Can you work these out from the model? Positions are in its coordinate system, mm. A direction names the side the tool comes from. Coordinates: 2 decimals unless noted, no trailing zeros. Loops run counter-clockwise (first coordinate to the right, second up) from the corner with the lowest first, then second, coordinate; pieces in that order, holes last. Notation, with made-up numbers: (83, -22.5) -> (92, -22.5) arc R9 cw to (92, -14.5) -> close; hole circle Ø4 at (70.5, 47.25). An arc over 180 degrees is marked (long way). Use one line per item in the form item = value. Start each with the question number.
(1) I need wall thicknesses on line 1 (X direction, y = -1.65, z = 0); line 2 (Z direction, x = -27.5, y = -5); line 3 (Z direction, x = -10.5, y = 11). Which ranges of each line are inside material? Lowest first, please. Write a range as [from, to].
(2) Imagine slicing it at B-B (z = 0). State how many separate pieces and enclosed holes the cut face has, plus the area to 3 significant figures.
(3) Imagine slicing it at A-A (x = -32.5). List the corners of the cut face in (y, z) for me, plus the area to 3 significant figures.
(4) Imagine slicing it at C-C (x = -49.5). List the corners of the cut face in (y, z) for me, plus the area to 3 significant figures.
(5) On a 3-axis mill with a long thin cutter (end or side, diameter ignored), from which of +Z, -Z, +X, -X, +Y, -Y can I reach the whole of each face in a straight line? I mean faces 5 (the flat face through (-8, 0, -1)), 6 (the cylindrical face through (-13.667, 13.133, -9.721)), 7 (the flat face through (-17.723, 10, -9)). Say none if no direction works.
(6) Thinking about a two-plate mould opening in Z: for faces 1 (the cylindrical face through (-38.7, 4.4, -1.5)), 2 (the cylindrical face through (-5.19, -2.96, -0.2)), 3 (the flat face through (-9.723, 6, -5)), 4 (the flat face through (-62.98, 8.83, -7.55)), which applies, released by +Z, released by -Z, zero draft, split by the parting line, or undercut?
(7) I'm going to push flat-ended pins straight in: pin 1 (5 mm diameter, centred on x = -10.5, z = 0, fed in from +Y); pin 2 (5 mm diameter, centred on x = -49.5, z = -6.5, fed in from -Y); pin 3 (1.8 mm diameter, centred on x = -21, y = -3.5, fed in from -Z). Where does each tip first touch, or does it pass through?
```python
from build123d import *

# Parameters (mm, degrees)
SKETCH_1_R          = 1.5
SKETCH_1_W          = 8
SKETCH_1_H          = 6
EXTRUDE_2_DEPTH     = 6
SKETCH_1_4_W        = 8
SKETCH_1_4_H        = 3
EXTRUDE_3_DEPTH     = 3
EXTRUDE_28_DEPTH    = 8
SKETCH_8_R          = 1.542364341
CUT_EXTRUDE_2_DEPTH = 12
EXTRUDE_29_DEPTH    = 35
EXTRUDE_30_DEPTH    = 8
CUT_EXTRUDE_START   = -20
SKETCH_11_R         = 1.5
CUT_EXTRUDE_3_DEPTH = 20


with BuildPart() as part:
    # Sketch 1 → Extrude 2 (new body)
    # profile 1 of 2: a face of its own
    with BuildSketch(Plane(origin=(0, 0, 0), x_dir=(1, 0, 0), z_dir=(0, 1, 0))):
        with BuildLine():
            Line((-38.676968887, 3), (-6.676968887, 3))
            ThreePointArc((-6.676968887, 3), (-3.676968887, 0), (-6.676968887, -3))
            Line((-6.676968887, -3), (-38.676968887, -3))
            ThreePointArc((-38.676968887, -3), (-41.676968887, 0), (-38.676968887, 3))
        make_face()
        with Locations(Location((-6.676968887, 0, 0), (0, 0, 270))):
            Circle(SKETCH_1_R, mode=Mode.SUBTRACT)
        with Locations(Location((-38.676968887, 0, 0), (0, 0, 270))):
            Circle(SKETCH_1_R, mode=Mode.SUBTRACT)
    # profile 2 of 2: a face of its own
    with BuildSketch(Plane(origin=(0, 0, 0), x_dir=(1, 0, 0), z_dir=(0, 1, 0))):
        with Locations((-13.722758256, 0)):
            Rectangle(SKETCH_1_W, SKETCH_1_H)
    extrude(amount=-EXTRUDE_2_DEPTH)

    # Sketch 1_4 → Extrude 3 (add)
    with BuildSketch(Plane(origin=(0, 0, 0), x_dir=(1, 0, 0), z_dir=(0, 1, 0))):
        with Locations((-13.722758256, -1.5)):
            Rectangle(SKETCH_1_4_W, SKETCH_1_4_H)
        with Locations((-13.722758256, 1.5)):
            Rectangle(SKETCH_1_4_W, SKETCH_1_4_H)
    extrude(amount=EXTRUDE_3_DEPTH)

    # Sketch 3 → Extrude 28 (add)
    with BuildSketch(Plane(origin=(-9.722758256, 0, 0), x_dir=(0, 0, -1), z_dir=(1, 0, 0))):
        with BuildLine():
            Line((3, -2.291502622), (12.260129589, 8.208497378))
            ThreePointArc((12.260129589, 8.208497378), (11.9058809, 13.854248689), (6.260129589, 13.5))
            Line((6.260129589, 13.5), (-3, 3))
            Line((-3, 3), (3, -2.291502622))
        make_face()
    extrude(amount=-EXTRUDE_28_DEPTH)

    # Sketch 8 → Cut-Extrude 2 (cut)
    with BuildSketch(Plane(origin=(-9.722758256, 0, 0), x_dir=(0, 0, -1), z_dir=(1, 0, 0))):
        with Locations((9.921567416, 11.604248689)):
            Circle(SKETCH_8_R)
    extrude(amount=-CUT_EXTRUDE_2_DEPTH, mode=Mode.SUBTRACT)

    # Sketch 9 → Extrude 29 (add)
    with BuildSketch(Plane.ZY.offset(17.722758256)):
        Polygon((-10.999130047, 6.778658296), (-4.999130047, 12.070160919), (2.276686058, 3.820160919), (-3.723313942, -1.471341704), align=None)
    extrude(amount=EXTRUDE_29_DEPTH)

    # Sketch 10 → Extrude 30 (add)
    with BuildSketch(Plane(origin=(0, -2.49076751, -2.824264888), x_dir=(-1, 0, 0), z_dir=(0, -0.6614378277661491, -0.7499999999999987))):
        with BuildLine():
            ThreePointArc((52.722758256, 6.859234408), (56.117999378, 11.940571837), (62.111845553, 10.748321705))
            Line((62.111845553, 10.748321705), (63.879612506, 12.516088658))
            ThreePointArc((63.879612506, 12.516088658), (58.113332077, 14.858485993), (52.413283237, 12.359234408))
            Line((52.413283237, 12.359234408), (52.722758256, 12.359234408))
            Line((52.722758256, 12.359234408), (52.722758256, 6.859234408))
        make_face()
        with BuildLine():
            Line((63.879612506, 1.202380159), (62.111845553, 2.970147112))
            ThreePointArc((62.111845553, 2.970147112), (56.117999378, 1.777896979), (52.722758256, 6.859234408))
            Line((52.722758256, 6.859234408), (52.722758256, 1.359234408))
            Line((52.722758256, 1.359234408), (52.413283237, 1.359234408))
            ThreePointArc((52.413283237, 1.359234408), (58.113332077, -1.140017176), (63.879612506, 1.202380159))
        make_face()
        with BuildLine():
            Line((52.722758256, 1.359234408), (52.722758256, 6.859234408))
            Line((52.722758256, 6.859234408), (52.722758256, 12.359234408))
            Line((52.722758256, 12.359234408), (52.413283237, 12.359234408))
            ThreePointArc((52.413283237, 12.359234408), (50.222758256, 6.859234408), (52.413283237, 1.359234408))
            Line((52.413283237, 1.359234408), (52.722758256, 1.359234408))
        make_face()
    extrude(amount=-EXTRUDE_30_DEPTH)

    # Sketch 11 → Cut-Extrude 3 (cut)
    with BuildSketch(Plane.XZ.offset(6).offset(CUT_EXTRUDE_START)):
        with Locations(Location((-38.676968887, 0, 0), (0, 0, 90))):
            Circle(SKETCH_11_R)
    extrude(amount=CUT_EXTRUDE_3_DEPTH, mode=Mode.SUBTRACT)


solid = part.part
```
Worked out:
q1.line_1 = [-41.68, -40.18], [-37.18, -8.18], [-5.18, -3.68]
q1.line_2 = [-3, 3]
q1.line_3 = [-13.26, -11.34], [-8.5, -4.06]
q2.separate_pieces = 4
q2.enclosed_holes = 0
q2.area = 429 mm2
q3.outline = (-6, -3) -> (-0.83, -3) -> (-1.47, -3.72) -> (6.78, -11) -> (12.07, -5) -> (3.82, 2.28) -> (0, -2.05) -> (0, 3) -> (-6, 3) -> close
q3.area = 124 mm2
q4.outline = (-1.47, -3.72) -> (6.78, -11) -> (12.07, -5) -> (3.82, 2.28) -> close
q4.area = 88.0 mm2
q5.face_5 = +Z, -Z, +X, +Y
q5.face_6 = +X
q5.face_7 = -Z, +Y
q6.face_1 = undercut
q6.face_2 = undercut
q6.face_3 = zero draft
q6.face_4 = released by +Z
q7.pin_1 = 9.24
q7.pin_2 = -1.16
q7.pin_3 = -3
